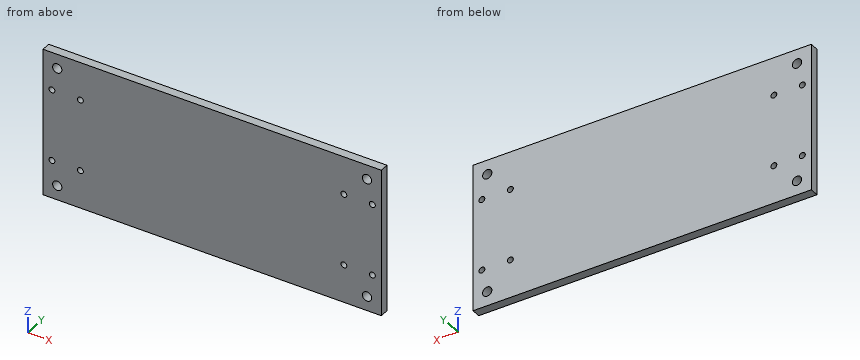
from build123d import *

# Parameters (mm, degrees)
SKETCH_1_W          = 347.5
SKETCH_1_H          = 165
SKETCH_1_R          = 2.6
EXTRUDE_1_DEPTH     = 5
SKETCH_2_W          = 157.5
SKETCH_2_H          = 82.5
SKETCH_2_H_2        = 55.334629905
SKETCH_2_H_3        = 27.165370095
SKETCH_2_R          = 2.6
SKETCH_2_W_2        = 173.75
SKETCH_2_W_3        = 16.25
CUT_EXTRUDE_2_DEPTH = 5
SKETCH_4_R          = 2.6
CUT_EXTRUDE_3_DEPTH = 5
SKETCH_5_R          = 1.65
CUT_EXTRUDE_4_DEPTH = 10


with BuildPart() as part:
    # 草图1 → 凸台-拉伸1 (new body)
    with BuildSketch(Plane(origin=(0, 5, 0), x_dir=(1, 0, 0), z_dir=(0, 1, 0))):
        Rectangle(SKETCH_1_W, SKETCH_1_H)
        with Locations(Location((-163.75, -70.5, 0), (0, 0, 90))):
            Circle(SKETCH_1_R, mode=Mode.SUBTRACT)
        with Locations(Location((-163.75, -60.5, 0), (0, 0, 90))):
            Circle(SKETCH_1_R, mode=Mode.SUBTRACT)
        with Locations(Location((163.75, -60.5, 0), (0, 0, 90))):
            Circle(SKETCH_1_R, mode=Mode.SUBTRACT)
        with Locations(Location((163.75, -70.5, 0), (0, 0, 90))):
            Circle(SKETCH_1_R, mode=Mode.SUBTRACT)
    extrude(amount=-EXTRUDE_1_DEPTH)

    # 草图2 → 切除-拉伸2 (cut)
    # profile 1 of 7: a face of its own
    with BuildSketch(Plane(origin=(0, 5, 0), x_dir=(1, 0, 0), z_dir=(0, 1, 0))):
        with Locations((-95, 41.25)):
            Rectangle(SKETCH_2_W, SKETCH_2_H)
    # profile 2 of 7: a face of its own
    with BuildSketch(Plane(origin=(0, 5, 0), x_dir=(1, 0, 0), z_dir=(0, 1, 0))):
        with Locations((-95, -27.667314952)):
            Rectangle(SKETCH_2_W, SKETCH_2_H_2)
    # profile 3 of 7: a face of its own
    with BuildSketch(Plane(origin=(0, 5, 0), x_dir=(1, 0, 0), z_dir=(0, 1, 0))):
        with Locations((-95, -68.917314952)):
            Rectangle(SKETCH_2_W, SKETCH_2_H_3)
        with Locations((-163.75, -70.5)):
            Circle(SKETCH_2_R, mode=Mode.SUBTRACT)
        with Locations((-163.75, -60.5)):
            Circle(SKETCH_2_R, mode=Mode.SUBTRACT)
    # profile 4 of 7: a face of its own
    with BuildSketch(Plane(origin=(0, 5, 0), x_dir=(1, 0, 0), z_dir=(0, 1, 0))):
        with Locations((86.875, -68.917314952)):
            Rectangle(SKETCH_2_W_2, SKETCH_2_H_3)
        with Locations((163.75, -70.5)):
            Circle(SKETCH_2_R, mode=Mode.SUBTRACT)
        with Locations((163.75, -60.5)):
            Circle(SKETCH_2_R, mode=Mode.SUBTRACT)
    # profile 5 of 7: a face of its own
    with BuildSketch(Plane(origin=(0, 5, 0), x_dir=(1, 0, 0), z_dir=(0, 1, 0))):
        with Locations((-8.125, -68.917314952)):
            Rectangle(SKETCH_2_W_3, SKETCH_2_H_3)
    # profile 6 of 7: a face of its own
    with BuildSketch(Plane(origin=(0, 5, 0), x_dir=(1, 0, 0), z_dir=(0, 1, 0))):
        with Locations((-8.125, -27.667314952)):
            Rectangle(SKETCH_2_W_3, SKETCH_2_H_2)
    # profile 7 of 7: a face of its own
    with BuildSketch(Plane(origin=(0, 5, 0), x_dir=(1, 0, 0), z_dir=(0, 1, 0))):
        with Locations((86.875, -27.667314952)):
            Rectangle(SKETCH_2_W_2, SKETCH_2_H_2)
    extrude(amount=-CUT_EXTRUDE_2_DEPTH, mode=Mode.SUBTRACT)

    # 草图4 → 切除-拉伸3 (cut)
    with BuildSketch(Plane(origin=(0, 5, 0), x_dir=(1, 0, 0), z_dir=(0, 1, 0))):
        with Locations(Location((165.75, 74.5, 0), (0, 0, 270))):
            Circle(SKETCH_4_R)
        with Locations(Location((165.75, 8, 0), (0, 0, 270))):
            Circle(SKETCH_4_R)
        with Locations(Location((-8.25, 74.5, 0), (0, 0, 270))):
            Circle(SKETCH_4_R)
        with Locations(Location((-8.25, 8, 0), (0, 0, 270))):
            Circle(SKETCH_4_R)
    extrude(amount=-CUT_EXTRUDE_3_DEPTH, mode=Mode.SUBTRACT)

    # 草图5 → 切除-拉伸4 (cut)
    with BuildSketch(Plane.XZ):
        with Locations(Location((-11.25, -61.25, 0), (0, 0, 270))):
            Circle(SKETCH_5_R)
        with Locations(Location((4.75, -61.25, 0), (0, 0, 270))):
            Circle(SKETCH_5_R)
        with Locations(Location((4.75, -21.25, 0), (0, 0, 270))):
            Circle(SKETCH_5_R)
        with Locations(Location((152.75, -61.25, 0), (0, 0, 270))):
            Circle(SKETCH_5_R)
        with Locations(Location((168.75, -61.25, 0), (0, 0, 270))):
            Circle(SKETCH_5_R)
        with Locations(Location((152.75, -21.25, 0), (0, 0, 270))):
            Circle(SKETCH_5_R)
        with Locations(Location((168.75, -21.25, 0), (0, 0, 270))):
            Circle(SKETCH_5_R)
        with Locations(Location((-11.25, -21.25, 0), (0, 0, 270))):
            Circle(SKETCH_5_R)
    extrude(amount=-CUT_EXTRUDE_4_DEPTH, mode=Mode.SUBTRACT)


solid = part.part
Could you check a few things on this model? Use its own coordinates, in mm. Give positions to 0.01 mm unless a question says otherwise; leave off trailing zeros. Order: outer loops, then holes, each group sorted by start corner. A loop starts at its lowest first (then second) coordinate and runs counter-clockwise, first axis right, second up. Notation, with made-up numbers: (-1.5, -30.75) - (47.5, -30.75) arc R29 ccw to (47.5, -8.75) - close; hole circle Ø6 at (72.5, 79). An arc over 180 degrees is marked (long way). One line per item, written item: value. Start each with the question number.
1. If I drill on probe 1 along Z at (x, y) = (152.75, 3.55); probe 2 along X at (y, z) = (3.6, -61.25); probe 3 along X at (y, z) = (1.95, -74.5), over which ranges is the centre line in solid material (lowest first)?
2. Imagine slicing it at B-B on z = -75. List the corners of the cut face in (x, y) for me, plus the area to 3 significant figures.
3. Imagine slicing it at A-A on z = -8. List the corners of the cut face in (x, y) for me, plus the area to 3 significant figures.
Values:
1. probe 1: -82.5 to -62.9, -59.6 to -22.9, -19.6 to 0
1. probe 2: -16.25 to -12.9, -9.6 to 3.1, 6.4 to 151.1, 154.4 to 167.1, 170.4 to 173.75
1. probe 3: -16.25 to -10.85, -5.65 to 163.15, 168.35 to 173.75
2. outline: (-16.25, 0) - (-10.8, 0) - (-10.8, 5) - (-16.25, 5) - close; (-5.7, 0) - (163.2, 0) - (163.2, 5) - (-5.7, 5) - close; (168.3, 0) - (173.75, 0) - (173.75, 5) - (168.3, 5) - close
2. area: 899 mm²
3. outline: (-16.25, 0) - (-10.85, 0) - (-10.85, 5) - (-16.25, 5) - close; (-5.65, 0) - (163.15, 0) - (163.15, 5) - (-5.65, 5) - close; (168.35, 0) - (173.75, 0) - (173.75, 5) - (168.35, 5) - close
3. area: 898 mm²
